from build123d import *

# Parameters (mm, degrees)
SKETCH2_W           = 6
SKETCH2_H           = 9.2
BOSS_EXTRUDE1_DEPTH = 6
SKETCH3_R           = 2.375
BOSS_EXTRUDE2_DEPTH = 3.2
SKETCH4_W           = 0.5
SKETCH4_H           = 0.5
BOSS_EXTRUDE3_DEPTH = 3.18


with BuildPart() as part:
    # Sketch2 → Boss-Extrude1 (new body)
    with BuildSketch(Plane(origin=(0, 0, 0), x_dir=(1, 0, 0), z_dir=(0, 1, 0))):
        with Locations((3, 4.6)):
            Rectangle(SKETCH2_W, SKETCH2_H)
    extrude(amount=BOSS_EXTRUDE1_DEPTH)

    # Sketch3 → Boss-Extrude2 (add)
    with BuildSketch(Plane.XY):
        with Locations((3, 3)):
            Circle(SKETCH3_R)
    extrude(amount=BOSS_EXTRUDE2_DEPTH)

    # Sketch4 → Boss-Extrude3 (add)
    with BuildSketch(Plane.XZ):
        with Locations((1.73, -5.75)):
            Rectangle(SKETCH4_W, SKETCH4_H)
        with Locations((4.27, -5.75)):
            Rectangle(SKETCH4_W, SKETCH4_H)
    extrude(amount=BOSS_EXTRUDE3_DEPTH)


solid = part.part
Geometry check sheet. Reference: the model listing, model coordinates, mm. A direction names the side the tool comes from. Coordinates: 2 decimals unless noted, no trailing zeros. Order: outer loops, then holes, each group sorted by start corner. A loop starts at its lowest first (then second) coordinate and runs counter-clockwise, first axis right, second up. Notation, with made-up numbers: (-2.5, 55.5) - (11.5, 55.5) arc R25 cw to (11.5, 89.5) - close; hole circle Ø8 at (-37, -17). An arc over 180 degrees is marked (long way). Answer in a Markdown table with one row per item. Add a question column.
1) Material ranges on line 1 along Z through (x, y) = (1.75, -0.75); line 2 along Y through (x, z) = (2.1, -5); line 3 along Z through (x, y) = (3.6, 5.5), recorded low to high. Write a range as [from, to].
2) Set-up check for faces 1 (the cylindrical face through (2.691, 5.355, 1.578)), 2 (the flat face through (3, 3, -9.2)): record each of +Z, -Z, +X, -X, +Y, -Y from which the full face is reachable in a straight line by a thin tool's end or side.
3) Cross-section at D-D, the plane z = 0.75. Record the cut outline in (x, y) (3 decimals), then the cut area to 3 significant figures.
4) Cross-section at A-A, the plane y = -2. Record the cut outline in (x, z), then the cut area to 3 significant figures.
5) Cross-section at B-B, the plane x = 3. Record the cut outline in (y, z) (3 decimals).
6) Cross-section at C-C, the plane y = 4. Record the cut outline in (x, z), then the cut area to 3 significant figures.
7) Gauge pin test, flat ends, axial feed: P1, Ø2, axis at y = -1.5, z = 0.5, coming from the -X side; P2, Ø0.6, axis at x = 4.5, y = -1.5, coming from the -Z side; P3, Ø2, axis at x = 4.5, y = -0.5, coming from the +Z side. Record the tip position at first contact, or that the pin passes through.
Check result:
| question | item | result |
|---|---|---|
| 1 | line 1 | z = [-6, -5.5] |
| 1 | line 2 | y = [0, 6] |
| 1 | line 3 | z = [-9.2, 0] |
| 2 | face 1 | +Z |
| 2 | face 2 | -Z, +X, -X, +Y, -Y |
| 3 | outline | circle Ø4.75 at (3, 3) |
| 3 | area | 17.7 mm² |
| 4 | outline | (1.48, -6) - (1.98, -6) - (1.98, -5.5) - (1.48, -5.5) - close; (4.02, -6) - (4.52, -6) - (4.52, -5.5) - (4.02, -5.5) - close |
| 4 | area | 0.500 mm² |
| 5 | outline | (0, -9.2) - (6, -9.2) - (6, 0) - (5.375, 0) - (5.375, 3.2) - (0.625, 3.2) - (0.625, 0) - (0, 0) - close |
| 6 | outline | (0, -9.2) - (6, -9.2) - (6, 0) - (5.15, 0) - (5.15, 3.2) - (0.85, 3.2) - (0.85, 0) - (0, 0) - close |
| 6 | area | 69.0 mm² |
| 7 | P1 | passes through |
| 7 | P2 | stops at z = -6 |
| 7 | P3 | stops at z = 0 |
